Autodesk Fusion 360 part; units mm, degrees
sketch "Sketch1" plane through (0, 0, 0) normal (0, 0, 1) x (1, 0, 0)
  line L0 (-156.1, 40) -> (50, 40)
  line L1 (50, 40) -> (50, 35)
  line L2 (50, 35) -> (-156.1, 35)
  line L3 (-156.1, 35) -> (-156.1, 40)
  circle A0 centre (-106.1, 25.5) radius 1.5
  circle A1 centre (0, 25.5) radius 1.5
  line L4 (-116.1, 35) -> (-96.1, 35)
  line L5 (-96.1, 35) -> (-96.1, 18)
  line L6 (-96.1, 18) -> (-116.1, 18)
  line L7 (-116.1, 18) -> (-116.1, 35)
  line L8 (-10, 35) -> (10, 35)
  line L9 (10, 35) -> (10, 18)
  line L10 (10, 18) -> (-10, 18)
  line L11 (-10, 18) -> (-10, 35)
  line L12 (-96.1, 18) -> (-86.285, 35)
  line L13 (-116.1, 18) -> (-125.915, 35)
  line L14 (-10, 18) -> (-19.815, 35)
  line L15 (10, 18) -> (19.815, 35)
  line L16 (50, 40) -> (45, 35)
  dimension "d1" = 206.1
  dimension "d2" = 5
  dimension "d3" = 3
  dimension "d4" = 3
  dimension "d5" = 50
  dimension "d6" = 14.5
  dimension "d7" = 50
  dimension "d8" = 14.5
  dimension "d9" = 10
  dimension "d10" = 10
  dimension "d11" = 7.5
  dimension "d12" = 10
  dimension "d13" = 10
  dimension "d14" = 7.5
  dimension "d15" = 30
  dimension "d16" = 30
  dimension "d17" = 30
  dimension "d18" = 30
  dimension "d19" = 45
extrude "Extrude1" add sketch "Sketch1" against normal blind 3.5 contours L2 L7 L13 | L2 L9 L15 | L2 L4 L5 L6 L7 | L2 L8 L9 L10 L11 | L2 L5 L12 | L2 L11 L14 makes body 1 at (-95.6839, 26.314, 0) makes body 2 at (10.4161, 26.314, 0)
extrude "Extrude2" add sketch "Sketch1" against normal blind 62.2 contours L0 L2 L3 L4 L8 L16 bodies 1 2
sketch "Sketch3" plane through (0, 0, 0) normal (0, 0, 1) x (-1, 0, 0)
  circle A0 centre (0, -25.5) radius 1.5
  circle A1 centre (106.1, -25.5) radius 1.5
  line L0 (96.1, -18) -> (86.285, -35)
  line L1 (86.285, -35) -> (19.815, -35)
  line L2 (19.815, -35) -> (10, -18)
  line L3 (10, -18) -> (-10, -18)
  line L4 (-10, -18) -> (-19.815, -35)
  line L5 (-19.815, -35) -> (-45, -35)
  line L6 (-45, -35) -> (-50, -40)
  line L7 (-50, -40) -> (156.1, -40)
  line L8 (125.915, -35) -> (116.1, -18)
  line L9 (116.1, -18) -> (96.1, -18)
  line L10 (-50, -40) -> (-26.5, -40)
  line L11 (-26.5, -40) -> (-26.5, -35)
  line L12 (-26.5, -35) -> (-50, -35)
  line L13 (-50, -35) -> (-50, -40)
  line L14 (156.1, -40) -> (132.6, -40)
  line L15 (132.6, -40) -> (132.6, -35)
  line L16 (132.6, -35) -> (156.1, -35)
  line L17 (156.1, -35) -> (156.1, -40)
  line L18 (156.1, -40) -> (156.1, -35)
  line L19 (156.1, -35) -> (125.915, -35)
  dimension "d28" = 5
  dimension "d29" = 23.5
  dimension "d30" = 5
  dimension "d31" = 23.5
extrude "Extrude3" cut sketch "Sketch3" against normal blind 4 contours L7 L14 L15 L16 L17 L18 L19 | L5 L6 L7 L10 L11 L12 bodies 1
sketch "Sketch4" plane through (0, 0, -62.2) normal (0, 0, -1) x (1, 0, 0)
  line L0 (45, -35) -> (-156.1, -35)
  line L1 (-156.1, -35) -> (-156.1, -40)
  line L2 (-156.1, -40) -> (50, -40)
  line L3 (50, -40) -> (45, -35)
  line L4 (50, -40) -> (48, -40)
  line L5 (48, -40) -> (48, -35)
  line L6 (48, -35) -> (50, -35)
  line L7 (50, -35) -> (50, -40)
  dimension "d34" = 5
  dimension "d35" = 2
extrude "Extrude5" cut sketch "Sketch4" against normal blind 22.4 contours L2 L3 L4 L5 bodies 1
sketch "Sketch5" plane through (0, 35, 0) normal (0, -1, 0) x (1, 0, 0)
  line L0 (-132.6, -4) -> (-156.1, -4)
  line L1 (-156.1, -4) -> (-156.1, -62.2)
  line L2 (-156.1, -62.2) -> (45, -62.2)
  line L3 (45, -62.2) -> (45, -4)
  line L4 (45, -4) -> (26.5, -4)
  line L5 (26.5, -4) -> (26.5, 0)
  line L6 (26.5, 0) -> (19.815, 0)
  line L7 (19.815, 0) -> (19.815, -3.5)
  line L8 (19.815, -3.5) -> (-19.815, -3.5)
  line L9 (-19.815, -3.5) -> (-19.815, 0)
  line L10 (-19.815, 0) -> (-86.285, 0)
  line L11 (-86.285, 0) -> (-86.285, -3.5)
  line L12 (-86.285, -3.5) -> (-125.915, -3.5)
  line L13 (-125.915, -3.5) -> (-125.915, 0)
  line L14 (-125.915, 0) -> (-132.6, 0)
  line L15 (-132.6, 0) -> (-132.6, -4)
  line L16 (-156.1, -4) -> (-151.1, -4)
  line L17 (-151.1, -4) -> (-151.1, -62.2)
  line L18 (-151.1, -62.2) -> (-156.1, -62.2)
  line L19 (-156.1, -62.2) -> (-156.1, -4)
  dimension "d40" = 5
extrude "Extrude6" add sketch "Sketch5" along normal blind 10 contours L0 L1 L2 L16 L17 L18 L19 bodies 1
fillet "Fillet1" radius 2 1 edges at (-156.1, 40, -33.1) on bodies 1
Could you check a few things on this model? Use its own coordinates, in mm. A direction names the side the tool comes from. Round coordinates to 2 decimals unless told otherwise and drop trailing zeros. Loops run counter-clockwise (first coordinate to the right, second up) from the corner with the lowest first, then second, coordinate; pieces in that order, holes last. Notation, with made-up numbers: (-22.5, 43.25) - (19.5, 43.25) arc R21 cw to (19.5, 74.25) - close; hole circle Ø3 at (83.5, -11.5). An arc over 180 degrees is marked (long way). Answer in a Markdown table with one row per item. Add a question column.
(1) I need wall thicknesses on line 1 along Y through (x, z) = (0, -1); line 2 along Y through (x, z) = (-36, -7); line 3 along Z through (x, y) = (-1, 34.5). Which ranges of each line are inside material? Lowest first, please.
(2) If we section it at D-D (z = -14.5): Please give me the cut outline in (x, y).
(3) If we section it at B-B (y = 30): Please give me the cut outline in (x, z), plus the area to 3 significant figures.
(4) If we section it at A-A (z = -44): Please give me the cut outline in (x, y), plus the area to 3 significant figures.
(5) If we section it at C-C (x = -55.5): Please give me the cut outline in (y, z).
(6) For faces 1 (the face through (-91.26, 26.38, -1.73)), 2 (the face through (26.5, 38, -2)), 3 (the face through (-132.6, 38, -2)), which set-ups out of +Z, -Z, +X, -X, +Y, -Y let a thin tool reach every point of the face, with its end or its side?
(7) I'm going to push flat-ended pins straight in: pin 1 (10 mm diameter, centred on x = -82, z = -13.5, fed in from -Y); pin 2 (2 mm diameter, centred on y = 37, z = -1, fed in from -X); pin 3 (2.5 mm diameter, centred on x = 35.5, y = 36.5, fed in from +Z). Where does each tip first touch, or does it pass through?
Model answer:
| question | item | result |
|---|---|---|
| 1 | line 1 | y = 18 to 24, 27 to 40 |
| 1 | line 2 | y = 35 to 40 |
| 1 | line 3 | z = -3.5 to 0 |
| 2 | outline | (-156.1, 25) - (-151.1, 25) - (-151.1, 35) - (45, 35) - (50, 40) - (-154.1, 40) arc R2 ccw to (-156.1, 38) - close |
| 3 | outline | (-156.1, -62.2) - (-151.1, -62.2) - (-151.1, -4) - (-156.1, -4) - close; (-123.03, -3.5) - (-89.17, -3.5) - (-89.17, 0) - (-123.03, 0) - close; (-16.93, -3.5) - (16.93, -3.5) - (16.93, 0) - (-16.93, 0) - close |
| 3 | area | 528 mm² |
| 4 | outline | (-156.1, 25) - (-151.1, 25) - (-151.1, 35) - (45, 35) - (48, 38) - (48, 40) - (-154.1, 40) arc R2 ccw to (-156.1, 38) - close |
| 4 | area | 1,070 mm² |
| 5 | outline | (35, -62.2) - (40, -62.2) - (40, 0) - (35, 0) - close |
| 6 | face 1 | +Z, -Z, -Y |
| 6 | face 2 | +Z, +X, +Y, -Y |
| 6 | face 3 | +Z, -X, +Y, -Y |
| 7 | pin 1 | stops at y = 35 |
| 7 | pin 2 | stops at x = -132.6 |
| 7 | pin 3 | stops at z = -4 |
